Part model, mm, in its own coordinate system. A direction names the side the tool comes from. Coordinates: 2 decimals unless noted, no trailing zeros. Write each loop counter-clockwise with the first axis right and the second up, starting at its lowest first coordinate (ties: lowest second). Pieces come first, ordered by that corner, then holes. Notation, with made-up numbers: (-30.5, 86) - (-11.5, 86) arc R31 cw to (-11.5, 116) - close; hole circle Ø3 at (-1.75, 27). An arc over 180 degrees is marked (long way). Write each question's results on one line, items separated by ' | '.
from build123d import *

# Parameters (mm, degrees)
BOX3522_W        = 1400
BOX3522_H        = 1000
BOX3522_DEPTH    = 500
ARRAY279_Z_COUNT = 4
ARRAY279_Z_PITCH = 550
BOX3520_W        = 500
BOX3520_H        = 500
BOX3520_DEPTH    = 2200
BOX3521_W        = 1500
BOX3521_H        = 600
BOX3521_DEPTH    = 2200


with BuildPart() as array279:
    # Box3522 → Box3522 (new body)
    with BuildSketch(Plane(origin=(7150, -2050, 0), x_dir=(1, 0, 0), z_dir=(0, 0, 1))):
        with Locations((700, 500)):
            Rectangle(BOX3522_W, BOX3522_H)
    extrude(amount=BOX3522_DEPTH)

    # Array279 Z: Array279 ×4


with BuildPart() as array279_1:
    add(array279.part)
    with Locations(*[(0, 0, i * ARRAY279_Z_PITCH) for i in range(1, ARRAY279_Z_COUNT)]):
        add(array279.part)


with BuildPart() as box3520:
    # Box3520 → Box3520 (new body)
    with BuildSketch(Plane(origin=(7100, -2100, 0), x_dir=(1, 0, 0), z_dir=(0, 0, 1))):
        with Locations((250, 250)):
            Rectangle(BOX3520_W, BOX3520_H)
    extrude(amount=BOX3520_DEPTH)


with BuildPart() as cut001:
    # Box3521 → Box3521 (new body)
    with BuildSketch(Plane(origin=(7100, -1600, 0), x_dir=(1, 0, 0), z_dir=(0, 0, 1))):
        with Locations((750, 300)):
            Rectangle(BOX3521_W, BOX3521_H)
    extrude(amount=BOX3521_DEPTH)

    # Fusion014: union Box3520
    add(box3520.part)

    # Cut001: cut Array279
    add(array279_1.part, mode=Mode.SUBTRACT)


solid = cut001.part
(1) Flat gauge pin, fed straight in: P1, Ø12, axis at x = 8237.5, y = -1409, coming from the -Z side. Where does the tip first touch, or does it go through?
Return value:
P1: stops at z = 500
(2) Two-plate mould, pull along Z, no slides. Class faces 6 (the flat face through (7840, -1050, 246)), 7 (the flat face through (7680, -1018, 0)), 8 (the flat face through (7685, -1432, 550)): released by +Z, released by -Z, zero draft, split by the parting line, or undercut.
Return value:
face 6: zero draft | face 7: released by -Z | face 8: undercut
(3) Saw through at B-B on z = 134. Write the cut outline in (x, y), then the cut area to 4 significant figures.
Return value:
outline: (7100, -2100) - (7600, -2100) - (7600, -2050) - (7150, -2050) - (7150, -1050) - (8550, -1050) - (8550, -1600) - (8600, -1600) - (8600, -1000) - (7100, -1000) - close | area: 177,500 mm^2
(4) Saw through at C-C on x = 7242. Write the cut outline in (y, z).
Return value:
outline: (-2100, 0) - (-2050, 0) - (-2050, 500) - (-1050, 500) - (-1050, 0) - (-1000, 0) - (-1000, 2200) - (-2100, 2200) - close; hole (-2050, 550) - (-1050, 550) - (-1050, 1050) - (-2050, 1050) - close; hole (-2050, 1100) - (-1050, 1100) - (-1050, 1600) - (-2050, 1600) - close; hole (-2050, 1650) - (-1050, 1650) - (-1050, 2150) - (-2050, 2150) - close
(5) Wall check: line 1 (Z direction, x = 8374, y = -1160.5); line 2 (Y direction, x = 7472.5, z = 1515); line 3 (X direction, y = -1108, z = 592.5). Give the ranges that are in metal, low to high. Write a range as from..to.
Return value:
line 1: z = 500..550, 1050..1100, 1600..1650, 2150..2200 | line 2: y = -2100..-2050, -1050..-1000 | line 3: x = 7100..7150, 8550..8600
(6) 3-axis set-ups, long thin cutter, end or side, ignore diameter. For faces 1 (the flat face through (7685, -1432, 500)), 2 (the flat face through (7150, -1557, 796)), 3 (the flat face through (8550, -1329, 246)), 4 (the flat face through (7372, -2050, 1346)), 5 (the flat face through (8550, -1329, 796)): which of +Z, -Z, +X, -X, +Y, -Y reach the whole face in a straight line?
Return value:
face 1: -Z | face 2: none | face 3: -Z, -Y | face 4: +X | face 5: -Y
(7) Saw through at A-A on y = -1183. Write the cut outline in (x, z), then the cut area to 3 significant figures.
Return value:
outline: (7100, 0) - (7150, 0) - (7150, 500) - (8550, 500) - (8550, 0) - (8600, 0) - (8600, 2200) - (7100, 2200) - close; hole (7150, 550) - (8550, 550) - (8550, 1050) - (7150, 1050) - close; hole (7150, 1100) - (8550, 1100) - (8550, 1600) - (7150, 1600) - close; hole (7150, 1650) - (8550, 1650) - (8550, 2150) - (7150, 2150) - close | area: 500,000 mm^2
(8) Saw through at D-D on y = -1794.5. Write the cut outline in (x, z).
Return value:
outline: (7100, 0) - (7150, 0) - (7150, 500) - (7600, 500) - (7600, 550) - (7150, 550) - (7150, 1050) - (7600, 1050) - (7600, 1100) - (7150, 1100) - (7150, 1600) - (7600, 1600) - (7600, 1650) - (7150, 1650) - (7150, 2150) - (7600, 2150) - (7600, 2200) - (7100, 2200) - close
